```python
from build123d import *

# Parameters (mm, degrees)
SKETCH2_W           = 28
SKETCH2_H           = 33.2
BOSS_EXTRUDE1_DEPTH = 3
SKETCH4_W           = 21
SKETCH4_H           = 5
SKETCH4_H_2         = 8.2
CUT_EXTRUDE1_DEPTH  = 3
BOSS_EXTRUDE2_DEPTH = 3


with BuildPart() as part:
    # Sketch2 → Boss-Extrude1 (new body)
    with BuildSketch(Plane.XY):
        Rectangle(SKETCH2_W, SKETCH2_H)
    extrude(amount=BOSS_EXTRUDE1_DEPTH)

    # Sketch4 → Cut-Extrude1 (cut)
    with BuildSketch(Plane.XY.offset(3)):
        Polygon((14, 1.6), (14, 6.6), (-11, 6.6), (-11, 1.6), (-7, 1.6), align=None)
        with Locations((3.5, -0.9)):
            Rectangle(SKETCH4_W, SKETCH4_H)
        Polygon((14, -8.4), (14, -3.4), (-7, -3.4), (-11, -3.4), (-11, -8.4), (-7, -8.4), align=None)
        with Locations((3.5, -12.5)):
            Rectangle(SKETCH4_W, SKETCH4_H_2)
    extrude(amount=-CUT_EXTRUDE1_DEPTH, mode=Mode.SUBTRACT)

    # Sketch5 → Boss-Extrude2 (add)
    with BuildSketch(Plane.XY.offset(3)):
        with BuildLine():
            Line((11, 29.751530772), (11, 35.6))
            Line((11, 35.6), (5.151530772, 35.6))
            ThreePointArc((5.151530772, 35.6), (7.196699141, 31.796699141), (11, 29.751530772))
        make_face()
        with BuildLine():
            Line((11, 16.6), (11, 29.751530772))
            ThreePointArc((11, 29.751530772), (7.196699141, 31.796699141), (5.151530772, 35.6))
            Line((5.151530772, 35.6), (5, 35.6))
            Line((5, 35.6), (5, 16.6))
            Line((5, 16.6), (11, 16.6))
        make_face()
        with BuildLine():
            Line((14, 16.6), (14, 29.751530772))
            ThreePointArc((14, 29.751530772), (12.5, 29.6), (11, 29.751530772))
            Line((11, 29.751530772), (11, 16.6))
            Line((11, 16.6), (14, 16.6))
        make_face()
        with BuildLine():
            Line((14, 29.751530772), (14, 35.6))
            Line((14, 35.6), (11, 35.6))
            Line((11, 35.6), (11, 29.751530772))
            ThreePointArc((11, 29.751530772), (12.5, 29.6), (14, 29.751530772))
        make_face()
        with BuildLine():
            Line((14, 38.6), (14, 35.6))
            Line((14, 35.6), (14, 29.751530772))
            ThreePointArc((14, 29.751530772), (18.309475019, 32.35658351), (20, 37.1))
            ThreePointArc((20, 37.1), (11.746182785, 44.562021148), (5.151530772, 35.6))
            Line((5.151530772, 35.6), (11, 35.6))
            Line((11, 35.6), (11, 38.6))
            Line((11, 38.6), (14, 38.6))
        make_face()
    extrude(amount=-BOSS_EXTRUDE2_DEPTH)


solid = part.part
```
Read the model definition and answer for the solid it produces. Units are mm, in the model's axes. A direction names the side the tool comes from. Give positions to 0.01 mm unless a question says otherwise; leave off trailing zeros. Order: outer loops, then holes, each group sorted by start corner. A loop starts at its lowest first (then second) coordinate and runs counter-clockwise, first axis right, second up. Notation, with made-up numbers: (-23, 48) -> (25, 48) arc R8 ccw to (25, 54) -> close; hole circle Ø6 at (57, -39). An arc over 180 degrees is marked (long way). One line per item, written item: value. Start each with the question number.
(1) Straight lines are drawn through the part: L1, parallel to Y at x = -9.5, z = 2; L2, parallel to Y at x = 2, z = 1.75; L3, parallel to Y at x = -12.5, z = 1.5. For each, find the intervals that lie inside material, in ascending order.
(2) Flat-ended cylindrical pins translate along their axes: P1, Ø0.9, axis at y = 5, z = 2, coming from the +X side; P2, Ø1.5, axis at y = -14.5, z = 1, coming from the +X side; P3, Ø0.9, axis at x = -8.5, z = 2, coming from the +Y side. Find the tip coordinate at first contact, or state that the pin passes through.
(3) The part is cut by section A-A (x = 12.5). Determine the outline of the cut face in (y, z), and give its area (3 significant figures).
(4) The part is cut by section C-C (y = 19). Determine the outline of the cut face in (x, z), and give its area (3 significant figures).
(5) A tool of negligible diameter and unlimited length cuts with its end or side. For faces 1 (the flat face through (-5, 16.6, 1)), 2 (the flat face through (3, 14, 0)), 3 (the flat face through (-7, -13, 2)), 4 (the flat face through (-11, -6, 2)), 5 (the flat face through (14, 37, 2)), from which of +Z, -Z, +X, -X, +Y, -Y can it reach the whole face along a straight path? Write none if from no direction.
(6) For a pull along X with two mould halves and no side action, classify faces 6 (the flat face through (-9, 1.6, 2)), 7 (the flat face through (11, 37, 2)), 8 (the flat face through (14, 18, 2)) as released by +X, released by -X, zero draft, split by the parting line, or undercut.
(7) The part is cut by section B-B (z = 1.45). Determine the outline of the cut face in (x, y).
(8) The part is cut by section D-D (x = 4). Determine the outline of the cut face in (y, z).
Taken from the geometry:
1. L1: -16.6 to -8.4, -3.4 to 1.6, 6.6 to 16.6
1. L2: 6.6 to 16.6
1. L3: -16.6 to 16.6
2. P1: x = -11
2. P2: x = -7
2. P3: y = 16.6
3. outline: (6.6, 0) -> (35.6, 0) -> (35.6, 3) -> (6.6, 3) -> close; (38.6, 0) -> (44.6, 0) -> (44.6, 3) -> (38.6, 3) -> close
3. area: 105 mm^2
4. outline: (5, 0) -> (14, 0) -> (14, 3) -> (5, 3) -> close
4. area: 27.0 mm^2
5. face 1: +Z, -Z, -X, +Y
5. face 2: -Z, +X, -X, +Y, -Y
5. face 3: +Z, -Z, +X, -Y
5. face 4: +Z, -Z, +X
5. face 5: +Z, -Z
6. face 6: zero draft
6. face 7: undercut
6. face 8: released by +X
7. outline: (-14, -16.6) -> (-7, -16.6) -> (-7, -8.4) -> (-11, -8.4) -> (-11, -3.4) -> (-7, -3.4) -> (-7, 1.6) -> (-11, 1.6) -> (-11, 6.6) -> (14, 6.6) -> (14, 29.75) arc R7.5 ccw (long way) to (5.15, 35.6) -> (5, 35.6) -> (5, 16.6) -> (-14, 16.6) -> close; hole (11, 35.6) -> (14, 35.6) -> (14, 38.6) -> (11, 38.6) -> close
8. outline: (6.6, 0) -> (16.6, 0) -> (16.6, 3) -> (6.6, 3) -> close
